from build123d import *

# Parameters (mm, degrees)
F0_W         = 14
F0_H         = 30.5
F0_R         = 4.525
F1_DEPTH     = 15
F3_DEPTH     = 14.001
F4_R         = 1.6
F4_R_2       = 1
F5_DEPTH     = 14.001
F6_R         = 12
F7_T1_DEPTH  = 10
F7_T3_DEPTH  = 11.5
F7_T5_DEPTH  = 8
F7_S9_W      = 2
F7_S9_H      = 2
F7_T10_DEPTH = 2
F7_S15_W     = 2
F7_S15_H     = 2
F7_T16_DEPTH = 2
F7_T22_DEPTH = 13
F7_T25_ANGLE = 90
F7_T29_DEPTH = 13
F7_T32_ANGLE = 90


# Not quite as in the source:
# - a fillet or chamfer that OpenCascade refuses, or shapes differently, is made with other operations: its cross-section is extruded or revolved along the edge and cut away or added


with BuildPart() as f1:
    # F0 (on Front) → F1 (new body)
    with BuildSketch(Plane.XZ):
        with Locations((0, 4.75)):
            Rectangle(F0_W, F0_H)
        Circle(F0_R, mode=Mode.SUBTRACT)
    extrude(amount=F1_DEPTH)

    # F2 (on face) → F3 (cut, through all)
    with BuildSketch(Plane.YZ.offset(7)):
        Polygon((-15, -10.5), (0, -10.5), (-5, -5.5), (-15, -5.5), align=None)
    extrude(amount=-F3_DEPTH, mode=Mode.SUBTRACT)

    # F4 (on face) → F5 (cut, through all)
    with BuildSketch(Plane.YZ.offset(7)):
        with Locations((-1.9, 8)):
            Circle(F4_R)
        with Locations((-7.5, 0)):
            Circle(F4_R_2)
    extrude(amount=-F5_DEPTH, mode=Mode.SUBTRACT)

    # F6
    f6_edges = [f1.edges().sort_by_distance(p)[0] for p in [
        (0, -15, 20),
    ]]
    fillet(f6_edges, radius=F6_R)

    # F7: fillet of radius 2 on 9 edges, made by hand

    # F7_s2 → F7_t1 (cut)
    with BuildSketch(Plane.YZ.offset(-5)):
        with BuildLine():
            ThreePointArc((-15, -3.5), (-14.4142135624, -4.9142135624), (-13, -5.5))
            Line((-13, -5.5), (-15, -5.5))
            Line((-15, -5.5), (-15, -3.5))
        make_face()
    extrude(amount=F7_T1_DEPTH, mode=Mode.SUBTRACT)

    # F7_s4 → F7_t3 (cut)
    with BuildSketch(Plane.XY.offset(-3.5)):
        with BuildLine():
            ThreePointArc((7, -13), (6.4142135624, -14.4142135624), (5, -15))
            Line((5, -15), (7, -15))
            Line((7, -15), (7, -13))
        make_face()
        with BuildLine():
            ThreePointArc((-7, -13), (-6.4142135624, -14.4142135624), (-5, -15))
            Line((-5, -15), (-7, -15))
            Line((-7, -15), (-7, -13))
        make_face()
    extrude(amount=F7_T3_DEPTH, mode=Mode.SUBTRACT)

    # F7_s6 → F7_t5 (cut)
    with BuildSketch(Plane.XZ.offset(-5)):
        with BuildLine():
            ThreePointArc((5, 20), (6.4142135624, 19.4142135624), (7, 18))
            Line((7, 18), (7, 20))
            Line((7, 20), (5, 20))
        make_face()
        with BuildLine():
            ThreePointArc((-5, 20), (-6.4142135624, 19.4142135624), (-7, 18))
            Line((-7, 18), (-7, 20))
            Line((-7, 20), (-5, 20))
        make_face()
    extrude(amount=F7_T5_DEPTH, mode=Mode.SUBTRACT)


with BuildPart() as f7_tool8:
    # F7_s9 → F7_t10 (new body)
    with BuildSketch(Plane.YZ.offset(5)):
        with Locations((-14, -4.5)):
            Rectangle(F7_S9_W, F7_S9_H)
    extrude(amount=F7_T10_DEPTH)

    # F7_s11 → F7_t12 (revolve, cut)
    with BuildSketch(Plane(origin=(5, -13, -3.5), x_dir=(0, 0.7071067812, 0.7071067812), z_dir=(0, 0.7071067812, -0.7071067812))):
        with BuildLine():
            ThreePointArc((0, -2), (2, 0), (0, 2))
            Line((0, 2), (0, -2))
        make_face()
    revolve(axis=Axis((5, -13, -3.5), (1, 0, 0)), mode=Mode.SUBTRACT)


with BuildPart() as f1_1:
    add(f1.part)

    # F7_t7: cut F7_tool8
    add(f7_tool8.part, mode=Mode.SUBTRACT)


with BuildPart() as f7_tool14:
    # F7_s15 → F7_t16 (new body)
    with BuildSketch(Plane.YZ.offset(-5)):
        with Locations((-14, -4.5)):
            Rectangle(F7_S15_W, F7_S15_H)
    extrude(amount=-F7_T16_DEPTH)

    # F7_s17 → F7_t18 (revolve, cut)
    with BuildSketch(Plane(origin=(-5, -13, -3.5), x_dir=(0, 0.7071067812, 0.7071067812), z_dir=(0, -0.7071067812, 0.7071067812))):
        with BuildLine():
            ThreePointArc((0, -2), (2, 0), (0, 2))
            Line((0, 2), (0, -2))
        make_face()
    revolve(axis=Axis((-5, -13, -3.5), (-1, 0, 0)), mode=Mode.SUBTRACT)


with BuildPart() as f1_2:
    add(f1_1.part)

    # F7_t13: cut F7_tool14
    add(f7_tool14.part, mode=Mode.SUBTRACT)


with BuildPart() as f7_tool20:
    # F7_s21 → F7_t22 (new body)
    with BuildSketch(Plane.XZ):
        with BuildLine():
            ThreePointArc((-7, -3.5), (-6.4142135624, -4.9142135624), (-5, -5.5))
            Line((-5, -5.5), (-7, -5.5))
            Line((-7, -5.5), (-7, -3.5))
        make_face()
    extrude(amount=F7_T22_DEPTH)

    split(bisect_by=Plane(origin=(0, -5.25, -5.25), x_dir=(1, 0, 0), z_dir=(0, -0.7071067812, -0.7071067812)), keep=Keep.TOP)


with BuildPart() as f1_3:
    add(f1_2.part)

    # F7_t19: cut F7_tool20
    add(f7_tool20.part, mode=Mode.SUBTRACT)

    # F7_s24 → F7_t25 (revolve, cut)
    with BuildSketch(Plane.XZ.offset(3)):
        with BuildLine():
            ThreePointArc((-5, 20), (-6.4142135624, 19.4142135624), (-7, 18))
            Line((-7, 18), (-7, 20))
            Line((-7, 20), (-5, 20))
        make_face()
    revolve(axis=Axis((-7, -3, 8), (1, 0, 0)), revolution_arc=F7_T25_ANGLE, mode=Mode.SUBTRACT)


with BuildPart() as f7_tool27:
    # F7_s28 → F7_t29 (new body)
    with BuildSketch(Plane.XZ):
        with BuildLine():
            ThreePointArc((7, -3.5), (6.4142135624, -4.9142135624), (5, -5.5))
            Line((5, -5.5), (7, -5.5))
            Line((7, -5.5), (7, -3.5))
        make_face()
    extrude(amount=F7_T29_DEPTH)

    split(bisect_by=Plane(origin=(0, -5.25, -5.25), x_dir=(1, 0, 0), z_dir=(0, -0.7071067812, -0.7071067812)), keep=Keep.TOP)


with BuildPart() as f1_4:
    add(f1_3.part)

    # F7_t26: cut F7_tool27
    add(f7_tool27.part, mode=Mode.SUBTRACT)

    # F7_s31 → F7_t32 (revolve, cut)
    with BuildSketch(Plane.XZ.offset(3)):
        with BuildLine():
            ThreePointArc((7, 18), (6.4142135624, 19.4142135624), (5, 20))
            Line((5, 20), (7, 20))
            Line((7, 20), (7, 18))
        make_face()
    revolve(axis=Axis((7, -3, 8), (1, 0, 0)), revolution_arc=F7_T32_ANGLE, mode=Mode.SUBTRACT)


solid = f1_4.part
Design review of the part built by this model. Coordinates are the model's own, in mm. A direction names the side the tool comes from. Round coordinates to 2 decimals unless told otherwise and drop trailing zeros. Write each loop counter-clockwise with the first axis right and the second up, starting at its lowest first coordinate (ties: lowest second). Pieces come first, ordered by that corner, then holes. Notation, with made-up numbers: (87.25, 48.5) - (99.25, 48.5) arc R3 ccw to (99.25, 52.5) - close; hole circle Ø2 at (41, 51.5). An arc over 180 degrees is marked (long way). Return JSON: item names as keys, results as strings. Group by question number.
Item 1: We need section C-C on x = 0.5. Write out the cut boundary in (y, z).
Item 2: The part is to be moulded in two halves that separate along Y. For faces 4 (the face through (-0.1, -2.8, -7.7)), 5 (the face through (5.7, -8.3, -0.6)), 6 (the face through (-7, -6, 7)), say which applies: pulls with the +Y half, pulls with the -Y half, needs draft (parallel to the pull), parting line crosses it, or undercut.
Item 3: We need section B-B on z = 0. Write out the cut boundary in (x, y) (3 decimals), and give its area (3 significant figures).
Item 4: Insertion check: P1, Ø5, axis at y = -1.9, z = 8, coming from the +X side; P2, Ø2, axis at x = 0.5, z = 1.5, coming from the -Y side; P3, Ø6.5, axis at x = 2.5, y = -7.5, coming from the -Z side. Each pin has a flat end and moves straight along its axis. Give the tip position at first contact, or say it passes through.
Item 5: Machinability: for faces 1 (the face through (6.43, -8.94, -4.9)), 2 (the face through (-6.43, -8.94, -4.9)), 3 (the face through (0, -9, -5.5)), which of the approach directions +Z, -Z, +X, -X, +Y, -Y give a long, thin tool a straight path to every point of the face, cutting with its end or side? Answer none if there is none.
Item 6: For probe 1 along Z at (x, y) = (3, -1.9); probe 2 along X at (y, z) = (-3.5, -3); probe 3 along Z at (x, y) = (-0.5, -2.75), list the stretches that pass through material, from the lowest coordinate up. Write a range as [from, to].
Item 7: We need section A-A on y = -1.9. Write out the cut boundary in (x, z) (3 decimals).
Item 8: We need section D-D on z = 7. Write out the cut boundary in (x, y), and give its area (3 significant figures).
Model answer:
{
 "1": {"outline": "(-15, 4.5) - (0, 4.5) - (0, 20) - (-3, 20) arc R12 ccw to (-15, 8) - close; (-14.73, -4.5) arc R2 ccw to (-13, -5.5) - (-5, -5.5) - (0, -10.5) - (0, -4.5) - close; hole circle Ø3.2 at (-1.9, 8)"},
 "2": {"face 4": "pulls with the -Y half", "face 5": "undercut", "face 6": "needs draft"},
 "3": {"outline": "(-7, -13) arc R2 ccw to (-5, -15) - (-4.525, -15) - (-4.525, -8.5) - (-7, -8.5) - close; (-7, -6.5) - (-4.525, -6.5) - (-4.525, 0) - (-7, 0) - close; (4.525, -15) - (5, -15) arc R2 ccw to (7, -13) - (7, -8.5) - (4.525, -8.5) - close; (4.525, -6.5) - (7, -6.5) - (7, 0) - (4.525, 0) - close", "area": "62.6 mm²"},
 "4": {"P1": "stops at x = 7", "P2": "passes through", "P3": "stops at z = -6.25"},
 "5": {"face 1": "-Z, +X, -Y", "face 2": "-Z, -X, -Y", "face 3": "-Z, +X, -X, -Y"},
 "6": {"probe 1": "z = [-8.6, -3.39], [3.39, 6.4], [9.6, 20]", "probe 2": "x = [-7, -3.39], [3.39, 7]", "probe 3": "z = [-7.75, -4.5], [4.5, 6.64], [9.36, 20]"},
 "7": {"outline": "(-7, -8.6) - (7, -8.6) - (7, 6.4) - (-7, 6.4) - close; (-7, 9.6) - (7, 9.6) - (7, 18) arc R2 ccw to (5, 20) - (-5, 20) arc R2 ccw to (-7, 18) - close; hole circle Ø9.05 at (0, 0)"},
 "8": {"outline": "(-7, -13) arc R2 ccw to (-5, -15) - (5, -15) arc R2 ccw to (7, -13) - (7, -3.15) - (-7, -3.15) - close; (-7, -0.65) - (7, -0.65) - (7, 0) - (-7, 0) - close", "area": "173 mm²"}
}
